Answer from the drawing. Dimensions are ordinates in mm from the lowest x, y and z of the part. A direction names the side the tool comes from. Round coordinates to 2 decimals unless told otherwise and drop trailing zeros. Loops run counter-clockwise (first coordinate to the right, second up) from the corner with the lowest first, then second, coordinate; pieces in that order, holes last. Notation, with made-up numbers: M 79,44 L 113,44 A30 ccw 113,70 Z; hole C 23,-0.5 d11. An arc over 180 degrees is marked long. One line per item, written item: value.
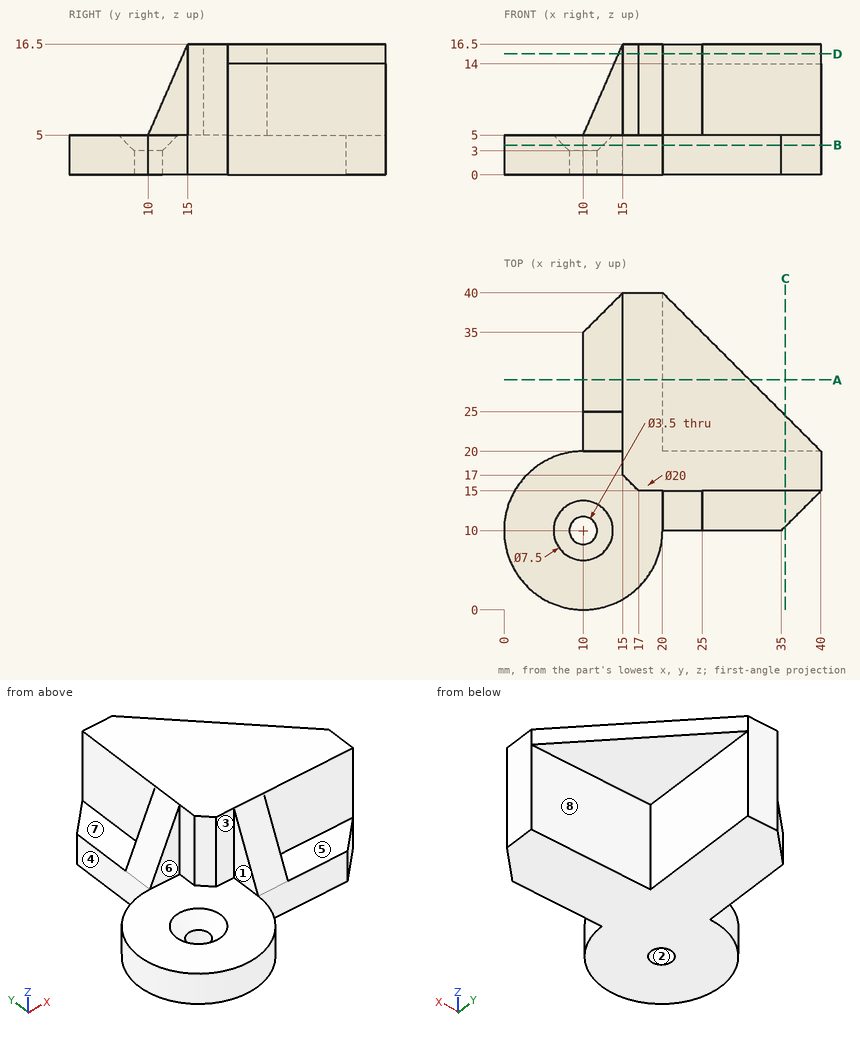
1) Find section A-A (y = 29). Give the vertices of the cut face in (x, z).
Check values:
outline: M 10,0 L 20,0 L 20,14 L 31,14 L 31,16.5 L 15,16.5 L 15,5 L 10,5 Z
2) Find section D-D (z = 15.25). Give the vertices of the cut face in (x, y).
Check values:
outline: M 14.46,20 L 15,20 L 15,17 L 17,15 L 20,15 L 20,14.46 L 25,14.46 L 25,15 L 40,15 L 40,20 L 20,40 L 15,40 L 15,25 L 14.46,25 Z
3) Find section C-C (x = 35.5). Give the vertices of the cut face in (y, z), then the cut area to 3 significant figures.
Check values:
outline: M 10.5,0 L 20,0 L 20,14 L 24.5,14 L 24.5,16.5 L 15,16.5 L 15,5 L 10.5,5 Z
area: 116 mm2
4) The mould has two halves that part along Y. Classify the marked faces 1, 2 and 3: +Y half, -Y half, draft (parallel to the pull), parting line (faces both ways), or undercut.
Check values:
face 1: draft
face 2: undercut
face 3: -Y half
5) For the marked faces 4, 5, 6, 7 and 8, determine the directions among +Z, -Z, +X, -X, +Y, -Y from which every point of the face is accessible in a straight line to the end or side of a thin tool.
Check values:
face 4: +Z, -Z, -X, +Y
face 5: +Z, +X, -Y
face 6: +Z, -X, -Y
face 7: +Z, -X, +Y
face 8: -Z, +X, +Y
6) Find the intervals of material crossed by probe 1 along X at (y, z) = (32, 12); probe 2 along Z at (x, y) = (35.5, 24); probe 3 along Y at (x, z) = (11.5, 6.5), in increasing order. Write a range as from..to.
Check values:
probe 1: 15..20
probe 2: 14..16.5
probe 3: 20..25
7) Each of these flat-tipped pins is pushed along its axis until it touches: pin 1 (1.5 mm diameter, centred on x = 22.5, y = 8, fed in from -Z); pin 2 (10 mm diameter, centred on x = 30.5, y = 8, fed in from +Z); pin 3 (6 mm diameter, centred on y = 28.5, z = 10.5, fed in from -X); pin 4 (3 mm diameter, centred on y = 20, z = 11, fed in from -X). Where does it stop, or does it pass through?
Check values:
pin 1: through
pin 2: z = 5
pin 3: x = 15
pin 4: x = 11.96
8) Find section B-B (z = 3.75). Give the vertices of the cut face in (x, y), then the cut area to 3 significant figures.
Check values:
outline: M 10,20 A10 ccw long 20,10 L 35,10 L 40,15 L 40,20 L 20,20 L 20,40 L 15,40 L 10,35 Z; hole C 10,10 d5
area: 691 mm2
